Verification items for the finished model (mm, model axes). Face numbers are marked on the shaded views. A direction names the side the tool comes from. Give positions to 0.01 mm unless a question says otherwise; leave off trailing zeros. Loops run counter-clockwise (first coordinate to the right, second up) from the corner with the lowest first, then second, coordinate; pieces in that order, holes last. Notation, with made-up numbers: M -9.75,78 L 26.25,78 A21 cw 26.25,86 Z; hole C -28.75,-1.5 d3. An arc over 180 degrees is marked long. Use a Markdown table: item, result.
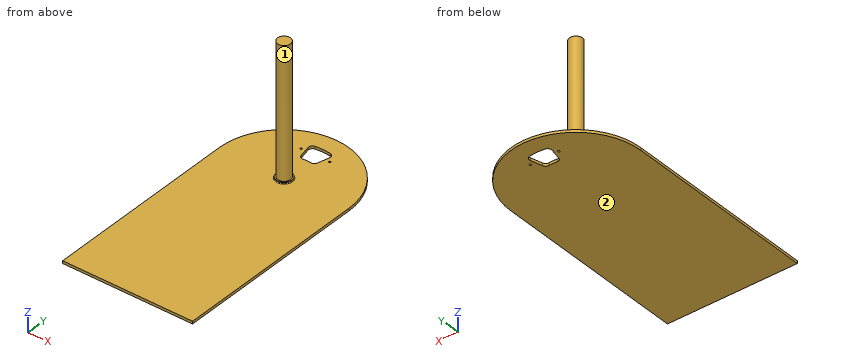
from build123d import *

# Parameters (mm, degrees)
SKETCH_1_R          = 50
EXTRUDE_1_DEPTH     = 2
SKETCH_2_R          = 6
EXTRUDE_2_DEPTH     = 1
SKETCH_3_R          = 5
EXTRUDE_3_DEPTH     = 100
FILLET_1_R          = 0.5
SKETCH_4_R          = 0.75
CUT_EXTRUDE_1_DEPTH = 10
SKETCH_5_W          = 100
SKETCH_5_H          = 150
EXTRUDE_4_DEPTH     = 2


with BuildPart() as part:
    # 草图1 → 凸台-拉伸1 (new body)
    with BuildSketch(Plane.XY):
        Circle(SKETCH_1_R)
        with BuildLine():
            Line((-8.46489845, 33.430105538), (-6.59071788, 24.612779199))
            ThreePointArc((-6.59071788, 24.612779199), (-5.371774848, 22.775404656), (-3.226125068, 22.267512592))
            ThreePointArc((-3.226125068, 22.267512592), (-0.282003378, 22.498232688), (2.666976337, 22.341379483))
            ThreePointArc((2.666976337, 22.341379483), (4.704329655, 22.835940411), (5.920350661, 24.543772946))
            Line((5.920350661, 24.543772946), (8.267408601, 33.303112428))
            ThreePointArc((8.267408601, 33.303112428), (7.884986755, 35.714496485), (5.836555568, 37.043010395))
            ThreePointArc((5.836555568, 37.043010395), (-0.088516087, 37.499895532), (-6.011364834, 37.015044142))
            ThreePointArc((-6.011364834, 37.015044142), (-8.006158275, 35.748212618), (-8.46489845, 33.430105538))
        make_face(mode=Mode.SUBTRACT)
    extrude(amount=EXTRUDE_1_DEPTH)

    # 草图2 → 凸台-拉伸2 (add)
    with BuildSketch(Plane.XY.offset(2)):
        Circle(SKETCH_2_R)
    extrude(amount=EXTRUDE_2_DEPTH)

    # 草图3 → 凸台-拉伸3 (add)
    with BuildSketch(Plane.XY.offset(3)):
        Circle(SKETCH_3_R)
    extrude(amount=EXTRUDE_3_DEPTH)

    # 圆角1
    fillet_1_edges = [part.edges().sort_by_distance(p)[0] for p in [
        (-6, 0, 2),
    ]]
    fillet(fillet_1_edges, radius=FILLET_1_R)

    # 草图4 → 切除-拉伸1 (cut)
    with BuildSketch(Plane(origin=(0, 0, 0), x_dir=(-1, 0, 0), z_dir=(0, 0, -1))):
        with Locations((-11, 30)):
            Circle(SKETCH_4_R)
        with Locations(Location((11, 30, 0), (0, 0, 180))):
            Circle(SKETCH_4_R)
    extrude(amount=-CUT_EXTRUDE_1_DEPTH, mode=Mode.SUBTRACT)

    # 草图5 → 凸台-拉伸4 (add)
    with BuildSketch(Plane.XY.offset(2)):
        with Locations((0, -75)):
            Rectangle(SKETCH_5_W, SKETCH_5_H)
    extrude(amount=-EXTRUDE_4_DEPTH)


solid = part.part
(1) Gauge pin test, flat ends, axial feed: P1, Ø1.5, axis at x = 30, y = -16, coming from the -Z side; P2, Ø1.5, axis at x = -0.5, y = -25, coming from the +Z side. Record the tip position at first contact, or that the pin passes through.
Results below:
| item | result |
|---|---|
| P1 | z = 0 |
| P2 | z = 2 |
(2) Set-up check for the marked faces 1 and 2: record each of +Z, -Z, +X, -X, +Y, -Y from which the full face is reachable in a straight line by a thin tool's end or side.
Results below:
| item | result |
|---|---|
| face 1 | +Z |
| face 2 | -Z, +X, -X, +Y, -Y |
(3) Material ranges on line 1 (Z direction, x = 9.5, y = -96.5); line 2 (Y direction, x = -11, z = 0.8) (3 decimals); line 3 (Y direction, x = -1, z = 42), recorded low to high.
Results below:
| item | result |
|---|---|
| line 1 | 0 to 2 |
| line 2 | -150 to 29.25, 30.75 to 48.775 |
| line 3 | -4.9 to 4.9 |
(4) Cross-section at A-A on x = 0. Record the cut outline in (y, z).
Results below:
| item | result |
|---|---|
| outline | M -150,0 L 22.5,0 L 22.5,2 L 6.5,2 A0.5 cw 6,2.5 L 6,3 L 5,3 L 5,103 L -5,103 L -5,3 L -6,3 L -6,2.5 A0.5 cw -6.5,2 L -150,2 Z; M 37.5,0 L 50,0 L 50,2 L 37.5,2 Z |
(5) Cross-section at B-B on y = -37. Record the cut outline in (x, z), then the cut area to 3 significant figures.
Results below:
| item | result |
|---|---|
| outline | M -50,0 L 50,0 L 50,2 L -50,2 Z |
| area | 200 mm^2 |
(6) Cross-section at C-C on z = 23.5. Record the cut outline in (x, y).
Results below:
| item | result |
|---|---|
| outline | C 0,0 d10 |
